Part model, mm, in its own coordinate system. A direction names the side the tool comes from. Give positions to 0.01 mm unless a question says otherwise; leave off trailing zeros. Loops run counter-clockwise (first coordinate to the right, second up) from the corner with the lowest first, then second, coordinate; pieces in that order, holes last. Notation, with made-up numbers: M -16,75.25 L 1,75.25 A13 cw 1,87.25 Z; hole C -22,53.5 d2. An arc over 180 degrees is marked long. Put each result on its own line as item: value. Start each with the question number.
```python
from build123d import *

# Parameters (mm, degrees)
F0_W     = 153.0927270651
F0_H     = 102.5236323476
F1_DEPTH = 25.4
F2_R     = 27.9986216142
F3_DEPTH = 50.8
F5_DEPTH = 121.412


# Not quite as in the source:
# - a feature names something its author has since deleted; it is built from what else it names


with BuildPart() as f1:
    # F0 (on Top) → F1 (new body)
    with BuildSketch(Plane.XY):
        with Locations((-0.1154541969, -0.3463625908)):
            Rectangle(F0_W, F0_H)
    extrude(amount=F1_DEPTH)

    # F2 (on face) → F3 (join)
    with BuildSketch(Plane.XY.offset(25.4)):
        Circle(F2_R)
    extrude(amount=F3_DEPTH)

    # F4 (on face) → F5 (cut)
    with BuildSketch(Plane.XZ.offset(51.6081787646)):
        Polygon((29.090275988, 49.3855252862), (29.2704553796, 77.5817409158), (-30.8739859611, 77.5817409158), align=None)
    extrude(amount=-F5_DEPTH, mode=Mode.SUBTRACT)


solid = f1.part
```
1) Band-saw the part on C-C on z = 46. Give the cut face in (x, y).
2) Pin check, flat tips, straight feed: pin 1 Ø10 at (x, z) = (23.5, 29) entering from -Y; pin 2 Ø1.5 at (x, y) = (35.5, 19) entering from +Z; pin 3 Ø3 at (y, z) = (-12.5, 45.5) entering from +X. Stop position of each tip, or through.
3) Wall check: L1, parallel to Z at x = -58.5, y = 25.5; L2, parallel to Y at x = 0.5, z = 47.5; L3, parallel to Y at x = -2, z = 36. Give the ranges that are in metal, low to high.
4) Which spindle directions (+Z, -Z, +X, -X, +Y, -Y) get a long thin tool onto all of the face, cutting with end or side? Do faces 1 (the flat face through (-1, 50.915, 13)), 2 (the cylindrical face through (-27.97, 1.23, 44.8)). Say none if no direction does.
5) Band-saw the part on B-B on x = 0. Give the cut face in (y, z), then the cut area to 3 significant figures.
6) Band-saw the part on A-A on y = 0. Give the cut face in (x, z), then the cut area to 3 significant figures.
7) Band-saw the part on D-D on y = 18.5. Give the cut face in (x, z), then the cut area to 3 significant figures.
Evaluation:
1. outline: C 0,0 d56
2. pin 1: y = -51.61
2. pin 2: z = 25.4
2. pin 3: x = 25.75
3. L1: 0 to 25.4
3. L2: -27.99 to 27.99
3. L3: -27.93 to 27.93
4. face 1: +Z, -Z, +X, -X, +Y
4. face 2: +Z
5. outline: M -51.61,0 L 50.92,0 L 50.92,25.4 L 28,25.4 L 28,63.06 L -28,63.06 L -28,25.4 L -51.61,25.4 Z
5. area: 4,710 mm2
6. outline: M -76.66,0 L 76.43,0 L 76.43,25.4 L 28,25.4 L 28,49.9 L -27.94,76.2 L -28,76.2 L -28,25.4 L -76.66,25.4 Z
6. area: 6,000 mm2
7. outline: M -76.66,0 L 76.43,0 L 76.43,25.4 L 21.02,25.4 L 21.02,53.18 L -21.02,72.95 L -21.02,25.4 L -76.66,25.4 Z
7. area: 5,470 mm2
